Design review of the part built by this model. Coordinates are the model's own, in mm. A direction names the side the tool comes from. Round coordinates to 2 decimals unless told otherwise and drop trailing zeros. Order: outer loops, then holes, each group sorted by start corner. A loop starts at its lowest first (then second) coordinate and runs counter-clockwise, first axis right, second up. Notation, with made-up numbers: (23, -10) - (77, -10) arc R10 ccw to (77, 3) - close; hole circle Ø8 at (22.25, 39). An arc over 180 degrees is marked (long way). Write item = value, one per line.
Autodesk Inventor part; units mm, degrees
ref_plane "Work Plane1" through (0, 0, -3.5) normal (0, 0, 1) x (1, 0, 0)
ref_plane "Work Plane2" through (0, 0, 3.5) normal (0, 0, 1) x (1, 0, 0)
ref_plane "YZ Plane" through (0, 0, 0) normal (1, 0, 0) x (0, 1, 0)
sketch "Sketch1" plane through (0, 0, 0) normal (0, 0, 1) x (1, 0, 0)
  line L0 (-8, 1.6) -> (8, 1.6)
  line L1 (8, 1.6) -> (8, 0)
  line L2 (8, 0) -> (-8, 0)
  line L3 (-8, 0) -> (-8, 1.6)
  arc A0 (-7.3, -8.3873) -> (-8.7, -8.3873) centre (-8, -8) ccw
  line L4 (-8.7, -8.3873) -> (-8.7, -10.4)
  line L5 (-7.3, -8.3873) -> (-7.3, -10.4)
  line L6 (-8, 0) -> (-10, -6.5)
  line L7 (-5.7087, -9) -> (2, 0)
  arc A1 (-7.3, -10.4) -> (-5.7087, -9) centre (-8, -8) ccw
  arc A2 (-10, -6.5) -> (-8.7, -10.4) centre (-8, -8) ccw
  point P0 (0, 0)
  point P1 (0, 0)
  dimension "d0" = 1.6
  dimension "d1" = 16
  dimension "d3" = 9.6
  dimension "d4" = 1.6
  dimension "d6" = 1.4
  dimension "d7" = 0.7
  dimension "d8" = 1
  dimension "d9" = 1.5
  dimension "d10" = 2.5
  dimension "d11" = 2.5
  dimension "d12" = 10
extrude "Extrusion1" add sketch "Sketch1" along normal mid plane 16 contours L0 L1 L2 L3
ref_plane "Work Plane1" through (0, 0, -3.5) normal (0, 0, 1) x (1, 0, 0)
ref_plane "Work Plane2" through (0, 0, 3.5) normal (0, 0, 1) x (1, 0, 0)
sketch "Sketch2" plane through (0, 0, 3.5) normal (0, 0, 1) x (1, 0, 0)
  line L0 (-8, 0) -> (-10, -6.5)
  arc A0 (-10, -6.5) -> (-8.7, -10.4) centre (-8, -8) ccw
  line L1 (-8.7, -8.3873) -> (-8.7, -10.4)
  arc A1 (-7.3, -8.3873) -> (-8.7, -8.3873) centre (-8, -8) ccw
  line L2 (-7.3, -8.3873) -> (-7.3, -10.4)
  arc A2 (-7.3, -10.4) -> (-5.7087, -9) centre (-8, -8) ccw
  line L3 (-5.7087, -9) -> (2, 0)
  line L4 (8, 0) -> (-8, 0)
  point P0 (0, 0)
extrude "Extrusion2" add sketch "Sketch2" along normal blind 1.6
sketch "Sketch3" plane through (0, 0, -3.5) normal (0, 0, 1) x (1, 0, 0)
  line L0 (-8, 0) -> (-10, -6.5)
  arc A0 (-10, -6.5) -> (-8.7, -10.4) centre (-8, -8) ccw
  line L1 (-8.7, -8.3873) -> (-8.7, -10.4)
  arc A1 (-7.3, -8.3873) -> (-8.7, -8.3873) centre (-8, -8) ccw
  line L2 (-7.3, -8.3873) -> (-7.3, -10.4)
  arc A2 (-7.3, -10.4) -> (-5.7087, -9) centre (-8, -8) ccw
  line L3 (-5.7087, -9) -> (2, 0)
  line L4 (8, 0) -> (-8, 0)
  point P0 (0, 0)
extrude "Extrusion3" add sketch "Sketch3" against normal blind 1.6
fillet "Fillet1" radius 0.5 4 edges at (-8.7, -10.4, 4.3) (-7.3, -10.4, 4.3) (-7.3, -10.4, -4.3) (-8.7, -10.4, -4.3)
sketch "Sketch4" plane through (-8, 1.6, 8) normal (0, 1, 0) x (1, 0, 0)
  line L0 (16, 16) -> (0, 16)
  line L1 (0, 0) -> (0, 16)
  circle A0 centre (4, 12) radius 2.5
  circle A1 centre (12, 12) radius 2.5
  circle A2 centre (12, 4) radius 2.5
  circle A3 centre (4, 4) radius 2.5
  circle A4 centre (4, 12) radius 1.5
  circle A5 centre (12, 12) radius 1.5
  circle A6 centre (12, 4) radius 1.5
  circle A7 centre (4, 4) radius 1.5
  point P0 (8, 8)
  dimension "d22" = 8
  dimension "d23" = 8
  dimension "d24" = 4
  dimension "d25" = 4
  dimension "d26" = 5
  dimension "d27" = 3
extrude "Extrusion4" add sketch "Sketch4" along normal blind 1.6
sketch "Sketch5" plane through (-8, 0, -8) normal (0, -1, 0) x (1, 0, 0)
  line L0 (0, 11.5) -> (10, 11.5)
  line L1 (10, 11.5) -> (10, 4.5)
  line L2 (10, 4.5) -> (0, 4.5)
  line L3 (0, 4.5) -> (0, 11.5)
  point P0 (8, 8)
extrude "Extrusion5" cut sketch "Sketch5" against normal blind 0.6
equation "\"d7\" = 0.5 * d6"
properties part number "2415" material "Steel"
1) We need section A-A on y = 2. Write out the cut boundary in (x, z), and give its area (3 significant figures).
Findings:
outline = circle Ø5 at (-4, -4); circle Ø5 at (-4, 4); circle Ø5 at (4, -4); circle Ø5 at (4, 4); hole circle Ø3 at (-4, -4); hole circle Ø3 at (-4, 4); hole circle Ø3 at (4, -4); hole circle Ø3 at (4, 4)
area = 50.3 mm^2
2) The part is to be moulded in two halves that separate along X. For faces 6 (the flat face through (4, 1.6, -4)), 7 (the flat face through (-2, 3.2, 4)), 8 (the cylindrical face through (-1.615, 2.389, 4.751)), 9 (the flat face through (-1.908, -4.563, 4.289)), say which applies: released by +X, released by -X, zero draft, split by the parting line, or undercut.
Findings:
face_6 = undercut
face_7 = zero draft
face_8 = undercut
face_9 = released by +X
3) For faces 1 (the flat face through (6, 3.2, 4)), 2 (the cylindrical face through (-10.48, -8.33, -4.29)), 3 (the flat face through (-8, 1, 0)), 4 (the flat face through (-6, -3, -3.5)), 5 (the cylindrical face through (5.43, 2.39, 4.45)), list the 3-axis set-ups (+Z, -Z, +X, -X, +Y, -Y) from which the entire face can be reached by the end or side of a thin tool; tool diameter is ignored.
Findings:
face_1 = +Z, -Z, +X, -X, +Y
face_2 = +Z, -Z, -X
face_3 = +Z, -Z, -X, +Y
face_4 = -X, -Y
face_5 = +Y
4) Clearance check with flat-ended pins moving along their axes: pin 1 Ø2.5 at (x, z) = (-4, 4) entering from +Y; pin 2 Ø0.8 at (y, z) = (0.5, 0) entering from -X; pin 3 Ø1 at (y, z) = (-8.5, -4) entering from -X; pin 4 Ø2.5 at (x, y) = (-8, -8) entering from +Z. State where each tip first meets the part, or that it passes through.
Findings:
pin_1 = 1.6
pin_2 = -8
pin_3 = -10.5
pin_4 = 5.1
5) We need section B-B on x = 4. Write out the cut boundary in (y, z).
Findings:
outline = (0, -8) - (1.6, -8) - (1.6, -6.5) - (3.2, -6.5) - (3.2, -5.5) - (1.6, -5.5) - (1.6, -2.5) - (3.2, -2.5) - (3.2, -1.5) - (1.6, -1.5) - (1.6, 1.5) - (3.2, 1.5) - (3.2, 2.5) - (1.6, 2.5) - (1.6, 5.5) - (3.2, 5.5) - (3.2, 6.5) - (1.6, 6.5) - (1.6, 8) - (0, 8) - close
6) To check wall thickness, follow L1, parallel to X at y = 2, z = 4; L2, parallel to Z at x = -4.5, y = -5.5. State the ranges of each line that lie inside material, in increasing order. Write a range as from..to.
Findings:
L1 = -6.5..-5.5, -2.5..-1.5, 1.5..2.5, 5.5..6.5
L2 = -5.1..-3.5, 3.5..5.1
